from build123d import *

# Parameters (mm, degrees)
SKETCH_1_W               = 132
SKETCH_1_H               = 60
EXTRUDE_1_DEPTH          = 50
CUT_EXTRUDE_1_DEPTH      = 154.37535656
CUT_EXTRUDE_1_DEPTH_BACK = 154.37535656
SKETCH_2_R               = 8
CUT_EXTRUDE_1_2_DEPTH    = 18
CUT_EXTRUDE_1_2_DRAFT    = -30


with BuildPart() as part:
    # 草图1 → 凸台-拉伸1 (new body)
    with BuildSketch(Plane(origin=(0, 0, 0), x_dir=(1, 0, 0), z_dir=(0, 1, 0))):
        with Locations((66, -30)):
            Rectangle(SKETCH_1_W, SKETCH_1_H)
    extrude(amount=EXTRUDE_1_DEPTH)

    # 草图2 → Cut-Extrude 1 (cut, two sides: drawn at the far end of the back side and taken through both)
    with BuildSketch(Plane(origin=(0, 50, 0), x_dir=(1, 0, 0), z_dir=(0, 1, 0)).offset(-CUT_EXTRUDE_1_DEPTH_BACK)):
        with Locations(Location((16, -30, 0), (0, 0, 270))):
            Circle(SKETCH_2_R)
        with Locations(Location((116, -30, 0), (0, 0, 270))):
            Circle(SKETCH_2_R)
    extrude(amount=CUT_EXTRUDE_1_DEPTH + CUT_EXTRUDE_1_DEPTH_BACK, mode=Mode.SUBTRACT)


with BuildPart() as cut_extrude_1_2_tool:
    # 草图4 → Cut-Extrude 1 2 (with draft: the straight prism first)
    with BuildSketch(Plane(origin=(0, 50, 0), x_dir=(1, 0, 0), z_dir=(0, 1, 0))):
        Polygon((76.145931536, 37.57326891), (9.744604929, -77.437202462), (53.045875119, -102.437202462), (119.447201725, 12.57326891), align=None)
    extrude(amount=-CUT_EXTRUDE_1_2_DEPTH)
    # Cut-Extrude 1 2: the draft: its side faces are tilted about the plane it starts from
    cut_extrude_1_2_sides = [cut_extrude_1_2_tool.faces().sort_by_distance(p)[0] for p in [
        (42.945268233, 41, 19.931966776),
        (31.395240024, 41, 89.937202462),
        (86.246538422, 41, 44.931966776),
        (97.79656663, 41, -25.07326891),
    ]]
    draft(cut_extrude_1_2_sides, Plane(origin=(0, 50, 0), x_dir=(1, 0, 0), z_dir=(0, 1, 0)), CUT_EXTRUDE_1_2_DRAFT)


with BuildPart() as part_1:
    add(part.part)

    # Cut-Extrude 1 2: cut by cut_extrude_1_2_tool
    add(cut_extrude_1_2_tool.part, mode=Mode.SUBTRACT)


solid = part_1.part
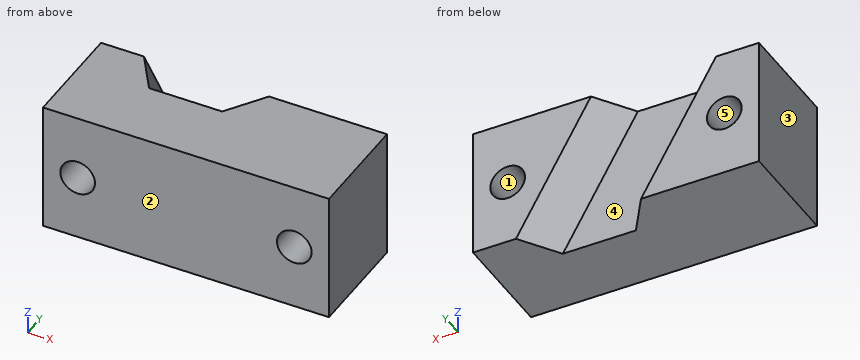
The listing builds one solid part. Answer for the finished solid, in the listing's coordinates (mm). Face numbers are marked on the shaded views. A direction names the side the tool comes from. Round coordinates to 2 decimals unless told otherwise and drop trailing zeros. Write each loop counter-clockwise with the first axis right and the second up, starting at its lowest first coordinate (ties: lowest second). Pieces come first, ordered by that corner, then holes. Notation, with made-up numbers: (63.25, 50.5) - (98.25, 50.5) arc R23 ccw to (98.25, 83.5) - close; hole circle Ø1 at (-24, 62.5). An arc over 180 degrees is marked (long way). Use a Markdown table: item, result. Add a question column.
1. For a pull along X with two mould halves and no side action, classify the marked faces 1, 2 and 3 as +X half, -X half, draft (parallel to the pull), parting line (faces both ways), or undercut.
2. Flat-ended cylindrical pins translate along their axes: P1, Ø9.5, axis at x = 16, z = 30, coming from the +Y side; P2, Ø18, axis at x = 79, z = 29.5, coming from the +Y side. Find the tip coordinate at first contact, or state that the pin passes through.
3. The part is cut by section D-D (z = 55.5). Write down the section's boundary in (x, y).
4. Consider line 1 (X direction, y = 28, z = 30); line 2 (Z direction, x = 16, y = 16); line 3 (X direction, y = 20.5, z = 36). Determine where each line is inside the solid, lowest interval first.
5. The part is cut by section B-B (z = 30). Write down the section's boundary in (x, y), and give its area (3 significant figures).
6. The part is cut by section C-C (x = 47.5). Write down the section's boundary in (y, z).
7. The part is cut by section A-A (x = 16). Write down the section's boundary in (y, z).
8. A tool of negligible diameter and unlimited length cuts with its end or side. For the marked faces 4 and 5, from which of +Z, -Z, +X, -X, +Y, -Y can it reach the whole face along a straight path? Write none if from no direction.
Reported:
| question | item | result |
|---|---|---|
| 1 | face 1 | undercut |
| 1 | face 2 | draft |
| 1 | face 3 | -X half |
| 2 | P1 | through |
| 2 | P2 | y = 41.35 |
| 3 | outline | (0, 0) - (132, 0) - (132, 50) - (80.15, 50) - (68.15, 32) - (34.41, 32) - (22.41, 50) - (0, 50) - close |
| 4 | line 1 | 0 to 8, 24 to 108, 124 to 132 |
| 4 | line 2 | 0 to 22, 38 to 60 |
| 4 | line 3 | 0 to 10.71, 21.29 to 110.71, 121.29 to 132 |
| 5 | outline | (0, 0) - (8, 0) - (8, 50) - (0, 50) - close; (24, 0) - (108, 0) - (108, 50) - (94.87, 50) - (82.87, 32) - (49.13, 32) - (37.13, 50) - (24, 50) - close; (124, 0) - (132, 0) - (132, 50) - (124, 50) - close |
| 5 | area | 4,180 mm^2 |
| 6 | outline | (0, 0) - (50, 0) - (50, 12.04) - (32, 32.83) - (32, 60) - (0, 60) - close |
| 7 | outline | (0, 0) - (50, 0) - (50, 22) - (0, 22) - close; (0, 38) - (50, 38) - (50, 60) - (0, 60) - close |
| 8 | face 4 | +Y |
| 8 | face 5 | +Y, -Y |
